Read the model definition and answer for the solid it produces. Units are mm, in the model's axes. A direction names the side the tool comes from. Round coordinates to 2 decimals unless told otherwise and drop trailing zeros. Loops run counter-clockwise (first coordinate to the right, second up) from the corner with the lowest first, then second, coordinate; pieces in that order, holes last. Notation, with made-up numbers: M 36,40.5 L 53,40.5 A38 cw 53,78.5 Z; hole C 50,17 d3. An arc over 180 degrees is marked long. Write each question's results on one line, items separated by ' | '.
Autodesk Inventor part; units mm, degrees
ref_plane "mirrored45" through (-12.5, 353.5534, -341.0534) normal (0, 0, 1) x (1, 0, 0)
ref_plane "YZ Plane" through (0, 0, 0) normal (1, 0, 0) x (0, 1, 0)
ref_plane "XZ Plane" through (0, 0, 0) normal (0, 1, 0) x (-1, 0, 0)
sketch "profile" plane through (0, 0, 0) normal (0, 1, 0) x (-1, 0, 0)
  line L0 (12.5, 12.5) -> (-12.5, 12.5)
  line L1 (-12.5, 12.5) -> (-12.5, -12.5)
  line L2 (-12.5, -12.5) -> (12.5, -12.5)
  line L3 (12.5, -12.5) -> (12.5, 12.5)
  line L4 (-10, -10) -> (-10, 10)
  line L5 (-10, 10) -> (10, 10)
  line L6 (10, 10) -> (10, -10)
  line L7 (10, -10) -> (-10, -10)
  point P0 (0, 0)
  dimension "d0" = 12.5
  dimension "d1" = 25
  dimension "d2" = 25
  dimension "d3" = 12.5
  dimension "d6" = 2.5
sketch3d "3D Sketch1"
  line L0 (0, 0, 0) -> (0, 353.5534, -353.5534)
  dimension "d4" = 500
  dimension "d5" = 45
sweep "Sweep1" add profiles "profile" path "3D Sketch1"
fillet "Fillet1" radius 2 4 edges at (-12.5, 176.7767, -189.2767) (-12.5, 176.7767, -164.2767) (12.5, 176.7767, -164.2767) (12.5, 176.7767, -189.2767)
ref_plane "mirrored45" through (-12.5, 353.5534, -341.0534) normal (0, 0, 1) x (1, 0, 0)
split "Split1" plane through (-12.5, 353.5534, -341.0534) removes the side toward (0, 0, -1)
equation "\"d1\" = width"
equation "\"d2\" = d1"
equation "\"d6\" = t"
equation "\"d4\" = L"
equation "\"d5\" = angleCut"
equation "\"d9\" = filletRadius"
equation "\"t\" = 2.5"
equation "\"filletRadius\" = 2"
equation "\"angleCut\" = 45deg"
equation "\"width\" = 25"
equation "\"a\" = 45"
properties part number "support_truss" material "Steel, Galvanized"
1. Find section A-A, the plane x = 0.5. Give the vertices of the cut face in (y, z), then the cut area to 3 significant figures.
Completed:
outline: M 0,-12.5 L 328.55,-341.05 L 331.05,-341.05 L 0,-10 Z; M 0,10 L 351.05,-341.05 L 353.55,-341.05 L 0,12.5 Z | area: 1,710 mm2
2. Which of the six approach directions +Z, -Z, +X, -X, +Y, -Y give full straight-line access (tool end or side, diameter ignored) to faces 1 (the face through (0, 0, -11)), 2 (the face through (10, 163, -166))?
Completed:
face 1: +Z, -Z, +X, -X, -Y | face 2: none
3. Determine the mould class of faces 3 (the face through (0, 178, -168)), 4 (the face through (-11.9, 167, -178.69)), 5 (the face through (-11.93, 178.83, -167.18)) for opening direction Z: released by +Z, released by -Z, zero draft, split by the parting line, or undercut.
Completed:
face 3: undercut | face 4: released by -Z | face 5: released by +Z
4. Given P1, Ø8, axis at x = -5, z = -223, coming from the -Y side; P2, Ø12, axis at x = -2.5, z = -203.5, coming from the -Y side; P3, Ø12, axis at y = 98, z = -116, coming from the -X side; P4, Ø8, axis at x = -4, z = -169.5, coming from the +Y side, each flat-ended and moving along its own axis, determine where each tip first touches the part or whether it passes through.
Completed:
P1: stops at y = 206.5 | P2: stops at y = 185 | P3: stops at x = -12.5 | P4: stops at y = 186
5. Find the intervals of material crossed by L1, parallel to Y at x = 6, z = -299.5; L2, parallel to Y at x = -1.75, z = -20.5; L3, parallel to Z at x = -6.25, y = 244.5, in increasing order.
Completed:
L1: y = 287 to 289.5, 309.5 to 312 | L2: y = 8 to 10.5, 30.5 to 33 | L3: z = -257 to -254.5, -234.5 to -232
